from build123d import *

# Parameters (mm, degrees)
CYLINDER019_R             = 1.7
CYLINDER019_DEPTH         = 20
PAD004_DEPTH              = 7.5
BOX003_W                  = 31.265144
BOX003_H                  = 19
BOX003_DEPTH              = 20
CYLINDER_R                = 56.1
CYLINDER_DEPTH            = 20
CYLINDER017_R             = 61.1
CYLINDER017_DEPTH         = 20
CYLINDER020_R             = 3.5
CYLINDER020_DEPTH         = 5
CYLINDER021_R             = 4
CYLINDER021_DEPTH         = 8
CYLINDER022_R             = 2.25
CYLINDER022_DEPTH         = 15
FUSION008_PLACEMENT_ANGLE = 90
CYLINDER023_R             = 4
CYLINDER023_DEPTH         = 8
CYLINDER024_R             = 2.25
CYLINDER024_DEPTH         = 15
FUSION009_PLACEMENT_ANGLE = 90
CYLINDER018_R             = 4.5
CYLINDER018_DEPTH         = 20
BOX005_W                  = 99.990908
BOX005_H                  = 15
BOX005_DEPTH              = 20
BOX004_W                  = 67.990908
BOX004_H                  = 38
BOX004_DEPTH              = 20


with BuildPart() as cylinder019:
    # Cylinder019 → Cylinder019 (new body)
    with BuildSketch(Plane(origin=(14.125764, 59, 0), x_dir=(1, 0, 0), z_dir=(0, 0, 1))):
        Circle(CYLINDER019_R)
    extrude(amount=CYLINDER019_DEPTH)


with BuildPart() as m8press002:
    # Sketch004 → Pad004 (new body)
    with BuildSketch(Plane.XY):
        Polygon((7.5, 0), (3.75, 6.495191), (-3.75, 6.495191), (-7.5, 0), (-3.75, -6.495191), (3.75, -6.495191), align=None)
    extrude(amount=PAD004_DEPTH)


with BuildPart() as m8press002_1:
    # Body004 placement: moved
    add(m8press002.part.moved(Location((-50.865144, 67, 0))))


with BuildPart() as cube003:
    # Box003 → Box003 (new body)
    with BuildSketch(Plane(origin=(-42.865144, 40, 0), x_dir=(1, 0, 0), z_dir=(0, 0, 1))):
        with Locations((15.632572, 9.5)):
            Rectangle(BOX003_W, BOX003_H)
    extrude(amount=BOX003_DEPTH)


with BuildPart() as cylinder:
    # Cylinder → Cylinder (new body)
    with BuildSketch(Plane.XY):
        Circle(CYLINDER_R)
    extrude(amount=CYLINDER_DEPTH)


with BuildPart() as common:
    # Cylinder017 → Cylinder017 (new body)
    with BuildSketch(Plane.XY):
        Circle(CYLINDER017_R)
    extrude(amount=CYLINDER017_DEPTH)

    # Cut: cut Cylinder
    add(cylinder.part, mode=Mode.SUBTRACT)

    # Common: intersect Cube003
    add(cube003.part, mode=Mode.INTERSECT)


with BuildPart() as cylinder020:
    # Cylinder020 → Cylinder020 (new body)
    with BuildSketch(Plane(origin=(14.125764, 59, 15), x_dir=(1, 0, 0), z_dir=(0, 0, 1))):
        Circle(CYLINDER020_R)
    extrude(amount=CYLINDER020_DEPTH)


with BuildPart() as cylinder021:
    # Cylinder021 → Cylinder021 (new body)
    with BuildSketch(Plane.XY):
        Circle(CYLINDER021_R)
    extrude(amount=CYLINDER021_DEPTH)


with BuildPart() as fusion008:
    # Cylinder022 → Cylinder022 (new body)
    with BuildSketch(Plane.XY):
        Circle(CYLINDER022_R)
    extrude(amount=CYLINDER022_DEPTH)

    # Fusion008: union Cylinder021
    add(cylinder021.part)


with BuildPart() as fusion008_1:
    # Fusion008 placement: moved
    add(fusion008.part.moved(Location((-68.865144, 52, 10))).rotate(Axis((-68.865144, 52, 10), (1, 0, 0)), FUSION008_PLACEMENT_ANGLE))


with BuildPart() as cylinder023:
    # Cylinder023 → Cylinder023 (new body)
    with BuildSketch(Plane.XY):
        Circle(CYLINDER023_R)
    extrude(amount=CYLINDER023_DEPTH)


with BuildPart() as fusion009:
    # Cylinder024 → Cylinder024 (new body)
    with BuildSketch(Plane.XY):
        Circle(CYLINDER024_R)
    extrude(amount=CYLINDER024_DEPTH)

    # Fusion009: union Cylinder023
    add(cylinder023.part)


with BuildPart() as fusion009_1:
    # Fusion009 placement: moved
    add(fusion009.part.moved(Location((15.125764, 52, 10))).rotate(Axis((15.125764, 52, 10), (1, 0, 0)), FUSION009_PLACEMENT_ANGLE))


with BuildPart() as fusion011:
    # Cylinder018 → Cylinder018 (new body)
    with BuildSketch(Plane(origin=(-50.865144, 67, 0), x_dir=(1, 0, 0), z_dir=(0, 0, 1))):
        Circle(CYLINDER018_R)
    extrude(amount=CYLINDER018_DEPTH)

    # Fusion011: union Cylinder019, M8Press002, Common, Cylinder020, Fusion008, Fusion009
    add(cylinder019.part)
    add(m8press002_1.part)
    add(common.part)
    add(cylinder020.part)
    add(fusion008_1.part)
    add(fusion009_1.part)


with BuildPart() as cube005:
    # Box005 → Box005 (new body)
    with BuildSketch(Plane(origin=(-76.865144, 37, 0), x_dir=(1, 0, 0), z_dir=(0, 0, 1))):
        with Locations((49.995454, 7.5)):
            Rectangle(BOX005_W, BOX005_H)
    extrude(amount=BOX005_DEPTH)


with BuildPart() as cut006:
    # Box004 → Box004 (new body)
    with BuildSketch(Plane(origin=(-60.865144, 37, 0), x_dir=(1, 0, 0), z_dir=(0, 0, 1))):
        with Locations((33.995454, 19)):
            Rectangle(BOX004_W, BOX004_H)
    extrude(amount=BOX004_DEPTH)

    # Fusion010: union Cube005
    add(cube005.part)

    # Cut006: cut Fusion011
    add(fusion011.part, mode=Mode.SUBTRACT)


solid = cut006.part
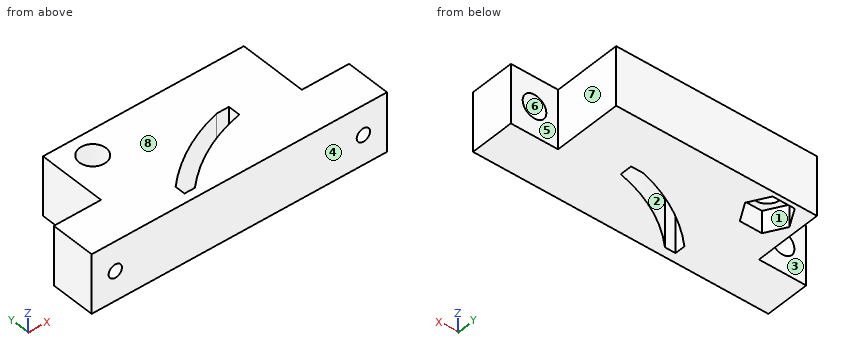
The model under review builds one solid part; all positions refer to its coordinate system, in mm. Face numbers are marked on the shaded views. A direction names the side the tool comes from. Coordinates: 2 decimals unless noted, no trailing zeros. Loops run counter-clockwise (first coordinate to the right, second up) from the corner with the lowest first, then second, coordinate; pieces in that order, holes last.
(1) Insertion check: P1, Ø10, axis at y = 68.5, z = 10, coming from the +X side; P2, Ø9, axis at x = 15.13, z = 10, coming from the +Y side; P3, Ø4.5, axis at y = 56.5, z = 6.5, coming from the -X side; P4, Ø3.5, axis at x = 15.13, z = 10, coming from the -Y side. Each pin has a flat end and moves straight along its axis. Give the tip position at first contact, or say it passes through.
Determined:
P1: stops at x = 7.13
P2: stops at y = 52
P3: stops at x = -60.87
P4: passes through
(2) Consider section C-C, the plane x = -25. Give the boundary of the cut face in (y, z), plus the area to 3 significant figures.
Determined:
outline: (37, 0) - (50.22, 0) - (50.22, 20) - (37, 20) - close; (55.75, 0) - (75, 0) - (75, 20) - (55.75, 20) - close
area: 649 mm2
(3) Draft analysis for pull direction Z (two halves, no side actions). For the marked faces 6, 7 and 8, state which applies: +Z half, -Z half, draft (parallel to the pull), parting line (faces both ways), or undercut.
Determined:
face 6: undercut
face 7: draft
face 8: +Z half
(4) Consider section A-A, the plane z = 10. Give the number of separate pieces and of enclosed holes in the cut face, plus the area to 3 significant figures.
Determined:
separate pieces: 3
enclosed holes: 2
area: 2,640 mm2
(5) Consider section B-B, the plane y = 49. Give the boundary of the cut face in (x, z), plus the area to 3 significant figures.
Determined:
outline: (-76.87, 0) - (-36.5, 0) - (-36.5, 20) - (-76.87, 20) - close; (-27.32, 0) - (23.13, 0) - (23.13, 20) - (-27.32, 20) - close; hole circle Ø8 at (-68.87, 10); hole circle Ø8 at (15.13, 10)
area: 1,720 mm2
(6) Wall thickness on L1, parallel to X at y = 39, z = 10; L2, parallel to Y at x = -50.5, z = 11.5; L3, parallel to X at y = 42.75, z = 10: over which ranges is each line inside the solid? List them lowest first.
Determined:
L1: x = -76.87 to -71.12, -66.62 to 12.88, 17.38 to 23.13
L2: y = 37 to 62.51, 71.49 to 75
L3: x = -76.87 to -71.12, -66.62 to -42.87, -36.33 to 12.88, 17.38 to 23.13
(7) Tool access review of the marked faces 1, 2, 3, 4 and 5: name each direction out of +Z, -Z, +X, -X, +Y, -Y from which nothing blocks a thin tool from reaching the whole face with its end or side.
Determined:
face 1: -Z
face 2: +Z, -Z
face 3: +Z, -Z, -X, +Y
face 4: +Z, -Z, +X, -X, -Y
face 5: +Z, -Z, +X, +Y
(8) Consider section D-D, the plane z = 3. Give the boundary of the cut face in (x, y), plus the area to 3 significant figures.
Determined:
outline: (-76.87, 37) - (23.13, 37) - (23.13, 52) - (7.13, 52) - (7.13, 75) - (-60.87, 75) - (-60.87, 52) - (-76.87, 52) - close; hole (-58.37, 67) - (-54.62, 60.5) - (-47.12, 60.5) - (-43.37, 67) - (-47.12, 73.5) - (-54.62, 73.5) - close; hole (-42.87, 40) - (-39.33, 40) arc R56.1 cw to (-11.6, 54.89) - (-11.6, 59) - (-15.88, 59) arc R61.1 ccw to (-42.87, 43.54) - close
area: 2,740 mm2
